For this review, use the dimensioned drawing (mm, ordinates from the lowest corner) and the shaded views. A direction names the side the tool comes from. Give positions to 0.01 mm unless a question says otherwise; leave off trailing zeros. Order: outer loops, then holes, each group sorted by start corner. A loop starts at its lowest first (then second) coordinate and runs counter-clockwise, first axis right, second up. Notation, with made-up numbers: (-35, 61.5) - (-19, 61.5) arc R29 ccw to (-19, 98.5) - close; hole circle Ø5 at (12, -11.5). An arc over 180 degrees is marked (long way). One line per item, written item: value.
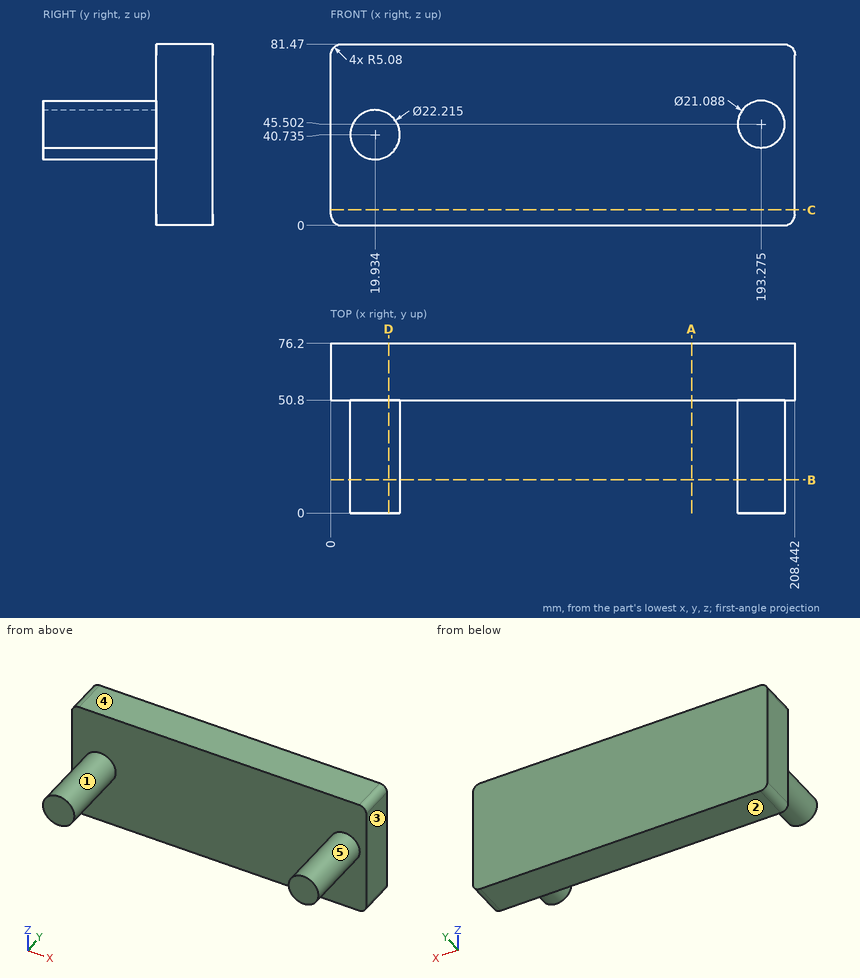
(1) For P1, Ø8, axis at x = 109, z = 67, coming from the -Y side, flat-tipped, find the tip position at first contact; note if it passes through.
Answers below:
P1: stops at y = 50.8
(2) Draft analysis for pull direction X (two halves, no side actions). For the marked faces 1, 2 and 3, state which applies: pulls with the +X half, pulls with the -X half, needs draft (parallel to the pull), parting line crosses it, or undercut.
Answers below:
face 1: undercut
face 2: needs draft
face 3: pulls with the +X half
(3) Machinability: for the marked faces 4 and 5, which of the approach directions +Z, -Z, +X, -X, +Y, -Y give a long, thin tool a straight path to every point of the face, cutting with its end or side? Answer none if there is none.
Answers below:
face 4: +Z, +X, -X, +Y, -Y
face 5: -Y
(4) Take a section at B-B (y = 15). Write out the cut boundary in (x, z) (1 decimal), then the cut area to 3 significant figures.
Answers below:
outline: circle Ø22.2 at (19.9, 40.7); circle Ø21.1 at (193.3, 45.5)
area: 737 mm^2
(5) Take a section at D-D (x = 26). Write out the cut boundary in (y, z).
Answers below:
outline: (0, 31.43) - (50.8, 31.43) - (50.8, 0) - (76.2, 0) - (76.2, 81.47) - (50.8, 81.47) - (50.8, 50.04) - (0, 50.04) - close
(6) Take a section at A-A (x = 162). Write out the cut boundary in (y, z), then the cut area to 3 significant figures.
Answers below:
outline: (50.8, 0) - (76.2, 0) - (76.2, 81.47) - (50.8, 81.47) - close
area: 2,070 mm^2
(7) Take a section at C-C (z = 7). Write out the cut boundary in (x, y), then the cut area to 3 significant figures.
Answers below:
outline: (0, 50.8) - (208.44, 50.8) - (208.44, 76.2) - (0, 76.2) - close
area: 5,290 mm^2
(8) Wall thickness on line 1 (Y direction, x = 39.5, z = 4.5); line 2 (Z direction, x = 14, y = 31) (1 decimal): over which ranges is each line inside the solid? List them lowest first. Write a range as from..to.
Answers below:
line 1: y = 50.8..76.2
line 2: z = 31.3..50.1
